```python
from build123d import *

# Parameters (mm, degrees)
SKETCH1_R           = 4.2
SKETCH1_R_2         = 4.25
SKETCH1_R_3         = 12.5
BOSS_EXTRUDE1_DEPTH = 10


with BuildPart() as part:
    # Sketch1 → Boss-Extrude1 (new body)
    with BuildSketch(Plane.XY):
        with BuildLine():
            Line((-80, -70), (80, -70))
            ThreePointArc((80, -70), (87.071067812, -67.071067812), (90, -60))
            Line((90, -60), (90, 180))
            ThreePointArc((90, 180), (87.071067812, 187.071067812), (80, 190))
            Line((80, 190), (-80, 190))
            ThreePointArc((-80, 190), (-87.071067812, 187.071067812), (-90, 180))
            Line((-90, 180), (-90, -60))
            ThreePointArc((-90, -60), (-87.071067812, -67.071067812), (-80, -70))
        make_face()
        with Locations((26.162950904, 26.162950904)):
            Circle(SKETCH1_R, mode=Mode.SUBTRACT)
        with Locations((26.162950904, -26.162950904)):
            Circle(SKETCH1_R, mode=Mode.SUBTRACT)
        with Locations((-26.162950904, -26.162950904)):
            Circle(SKETCH1_R, mode=Mode.SUBTRACT)
        with Locations((-26.162950904, 26.162950904)):
            Circle(SKETCH1_R, mode=Mode.SUBTRACT)
        with Locations((0, 63.5)):
            Circle(SKETCH1_R, mode=Mode.SUBTRACT)
        with Locations((-67.5, 167.5)):
            Circle(SKETCH1_R_2, mode=Mode.SUBTRACT)
        with Locations((-67.5, 122.5)):
            Circle(SKETCH1_R_2, mode=Mode.SUBTRACT)
        with Locations((-22.5, 122.5)):
            Circle(SKETCH1_R_2, mode=Mode.SUBTRACT)
        with Locations((-22.5, 167.5)):
            Circle(SKETCH1_R_2, mode=Mode.SUBTRACT)
        with Locations((22.5, 122.5)):
            Circle(SKETCH1_R_2, mode=Mode.SUBTRACT)
        with Locations((22.5, 167.5)):
            Circle(SKETCH1_R_2, mode=Mode.SUBTRACT)
        with Locations((67.5, 122.5)):
            Circle(SKETCH1_R_2, mode=Mode.SUBTRACT)
        with Locations((67.5, 167.5)):
            Circle(SKETCH1_R_2, mode=Mode.SUBTRACT)
        Circle(SKETCH1_R_3, mode=Mode.SUBTRACT)
    extrude(amount=BOSS_EXTRUDE1_DEPTH)


solid = part.part
```
Geometry check sheet. Reference: the model listing, model coordinates, mm. Round coordinates to 2 decimals unless told otherwise and drop trailing zeros. Write each loop counter-clockwise with the first axis right and the second up, starting at its lowest first coordinate (ties: lowest second). Pieces come first, ordered by that corner, then holes. Notation, with made-up numbers: (80.25, -5) -> (122.25, -5) arc R17 ccw to (122.25, 8) -> close; hole circle Ø5 at (60, 58). An arc over 180 degrees is marked (long way). Put each result on its own line as item: value.
1) Depth check by flat-ended pin: P1, Ø8, axis at x = -51.5, y = 153.5, coming from the -Z side; P2, Ø5, axis at x = 22.5, y = 122.5, coming from the +Z side. Enter the tip coordinate at first touch or a pass-through.
Recorded:
P1: stops at z = 0
P2: passes through
2) Thickness scan on probe 1 along X at (y, z) = (26, 6.5); probe 2 along Y at (x, z) = (-0.5, 0.5); probe 3 along Y at (x, z) = (-67.5, 3.5). Record the ranges inside material, lowest first. Write a range as from..to.
Recorded:
probe 1: x = -90..-30.36, -21.97..21.97, 30.36..90
probe 2: y = -70..-12.49, 12.49..59.33, 67.67..190
probe 3: y = -70..118.25, 126.75..163.25, 171.75..190
3) Cross-section at D-D, the plane y = 0. Enter the section's corners in (x, z).
Recorded:
outline: (-90, 0) -> (-12.5, 0) -> (-12.5, 10) -> (-90, 10) -> close; (12.5, 0) -> (90, 0) -> (90, 10) -> (12.5, 10) -> close
4) Cross-section at A-A, the plane y = 63.5. Enter the section's corners in (x, z).
Recorded:
outline: (-90, 0) -> (-4.2, 0) -> (-4.2, 10) -> (-90, 10) -> close; (4.2, 0) -> (90, 0) -> (90, 10) -> (4.2, 10) -> close
5) Cross-section at C-C, the plane y = 122.5. Enter the section's corners in (x, z), plus the area to 3 significant figures.
Recorded:
outline: (-90, 0) -> (-71.75, 0) -> (-71.75, 10) -> (-90, 10) -> close; (-63.25, 0) -> (-26.75, 0) -> (-26.75, 10) -> (-63.25, 10) -> close; (-18.25, 0) -> (18.25, 0) -> (18.25, 10) -> (-18.25, 10) -> close; (26.75, 0) -> (63.25, 0) -> (63.25, 10) -> (26.75, 10) -> close; (71.75, 0) -> (90, 0) -> (90, 10) -> (71.75, 10) -> close
area: 1,460 mm2
6) Cross-section at B-B, the plane x = 0. Enter the section's corners in (y, z), plus the area to 3 significant figures.
Recorded:
outline: (-70, 0) -> (-12.5, 0) -> (-12.5, 10) -> (-70, 10) -> close; (12.5, 0) -> (59.3, 0) -> (59.3, 10) -> (12.5, 10) -> close; (67.7, 0) -> (190, 0) -> (190, 10) -> (67.7, 10) -> close
area: 2,270 mm2
7) Release check for a two-part mould opening along Y. For faces 1 (the face through (-0.91, 59.4, 4.93)), 2 (the face through (1, 190, 5)), 3 (the face through (86.99, -67.15, 4.93)) record: pulls with the +Y half, pulls with the -Y half, needs draft (parallel to the pull), parting line crosses it, or undercut.
Recorded:
face 1: undercut
face 2: pulls with the +Y half
face 3: pulls with the -Y half
